Part print with two shaded views. Sizes in mm from the minimum x, y, z corner. Coordinates: 2 decimals unless noted, no trailing zeros. Write each loop counter-clockwise with the first axis right and the second up, starting at its lowest first coordinate (ties: lowest second). Pieces come first, ordered by that corner, then holes.
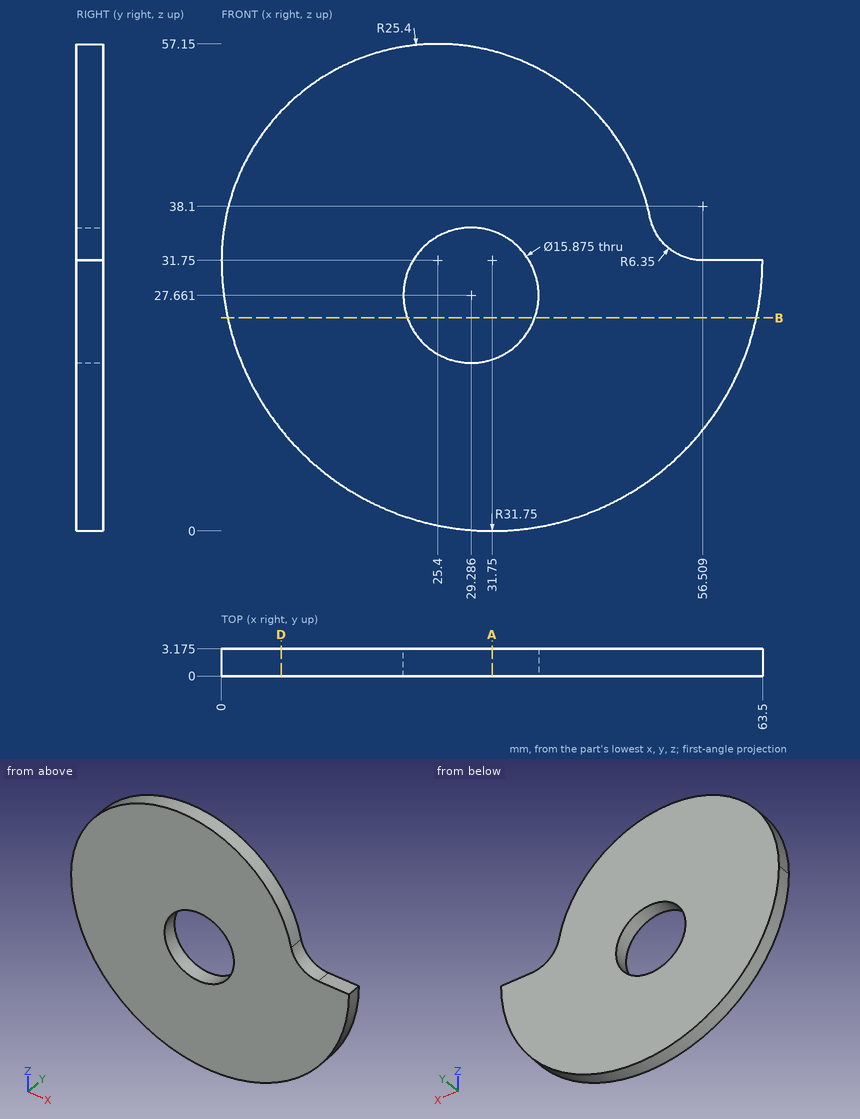
(1) Slice it at A-A, the plane x = 31.75. List the corners of the cut face in (y, z) (1 decimal).
(2) Slice it at B-B, the plane z = 25. List the corners of the cut face in (x, y) (1 decimal).
(3) Probe L1, parallel to Z at x = 24.5, y = 2.8 (1 decimal); L2, parallel to Z at x = 31.5, y = 1.9; L3, parallel to X at y = 3, z = 22.5 (1 decimal). List the from-to ranges inside material, lowest first.
(4) Slice it at D-D, the plane x = 7. List the corners of the cut face in (y, z) (1 decimal), and give its area (3 significant figures).
(5) Flat gauge pins, fed straight in: P1, Ø1.5, axis at x = 17.5, y = 0.5, coming from the +Z side; P2, Ø1.6, axis at x = 61.5, y = 1.5, coming from the +Z side; P3, Ø1.5, axis at x = 41, y = 0.5, coming from the -Z side. Where does each tip first touch, or does it go through?
Results:
1. outline: (0, 0) - (3.2, 0) - (3.2, 20.1) - (0, 20.1) - close; (0, 35.2) - (3.2, 35.2) - (3.2, 56.3) - (0, 56.3) - close
2. outline: (0.7, 0) - (21.8, 0) - (21.8, 3.2) - (0.7, 3.2) - close; (36.8, 0) - (62.8, 0) - (62.8, 3.2) - (36.8, 3.2) - close
3. L1: z = 0.8 to 21.3, 34 to 57.1
3. L2: z = 0 to 20.04, 35.28 to 56.41
3. L3: x = 1.4 to 23.3, 35.3 to 62.1
4. outline: (0, 11.9) - (3.2, 11.9) - (3.2, 49.3) - (0, 49.3) - close
4. area: 119 mm2
5. P1: stops at z = 56.12
5. P2: stops at z = 31.75
5. P3: stops at z = 1.16
